Part print with two shaded views. Sizes in mm from the minimum x, y, z corner. A direction names the side the tool comes from. Give positions to 0.01 mm unless a question says otherwise; leave off trailing zeros. Loops run counter-clockwise (first coordinate to the right, second up) from the corner with the lowest first, then second, coordinate; pieces in that order, holes last. Notation, with made-up numbers: (-21, -10) -> (-11, -10) arc R11 cw to (-11, 1) -> close; hole circle Ø3 at (50.5, 51.25). An arc over 180 degrees is marked (long way). One line per question, with ' | ' between items. Start each with the question number.
(1) Slice it at D-D, the plane x = 16. Write the cut outline in (y, z).
(2) Flat gauge pins, fed straight in: pin 1 Ø2 at (x, y) = (32.5, 10) entering from +Z; pin 2 Ø2 at (x, z) = (25.72, 20.32) entering from -Y; pin 3 Ø12.5 at (x, z) = (23.5, 15) entering from -Y. Where does each tip first touch, or does it go through?
(3) Slice it at B-B, the plane z = 20.32. Write the cut outline in (x, y) (1 decimal).
(4) Drill centre lines: L1, parallel to X at y = 23.6, z = 20.32 (1 decimal); L2, parallel to X at y = 18.75, z = 1.5; L3, parallel to Y at x = 18.5, z = 13. Where is each one in solid material? Low to high. Write a range as from..to.
(5) 3-axis set-ups, long thin cutter, end or side, ignore diameter. For the marked faces 1, 2 and 3: which of +Z, -Z, +X, -X, +Y, -Y reach the whole face in a straight line?
(6) Slice it at C-C, the plane x = 29. Write the cut outline in (y, z) (1 decimal).
(7) Mould opens along X. For the marked faces 4, 5, 6 and 7 say: pulls with the +X half, pulls with the -X half, needs draft (parallel to the pull), parting line crosses it, or undercut.
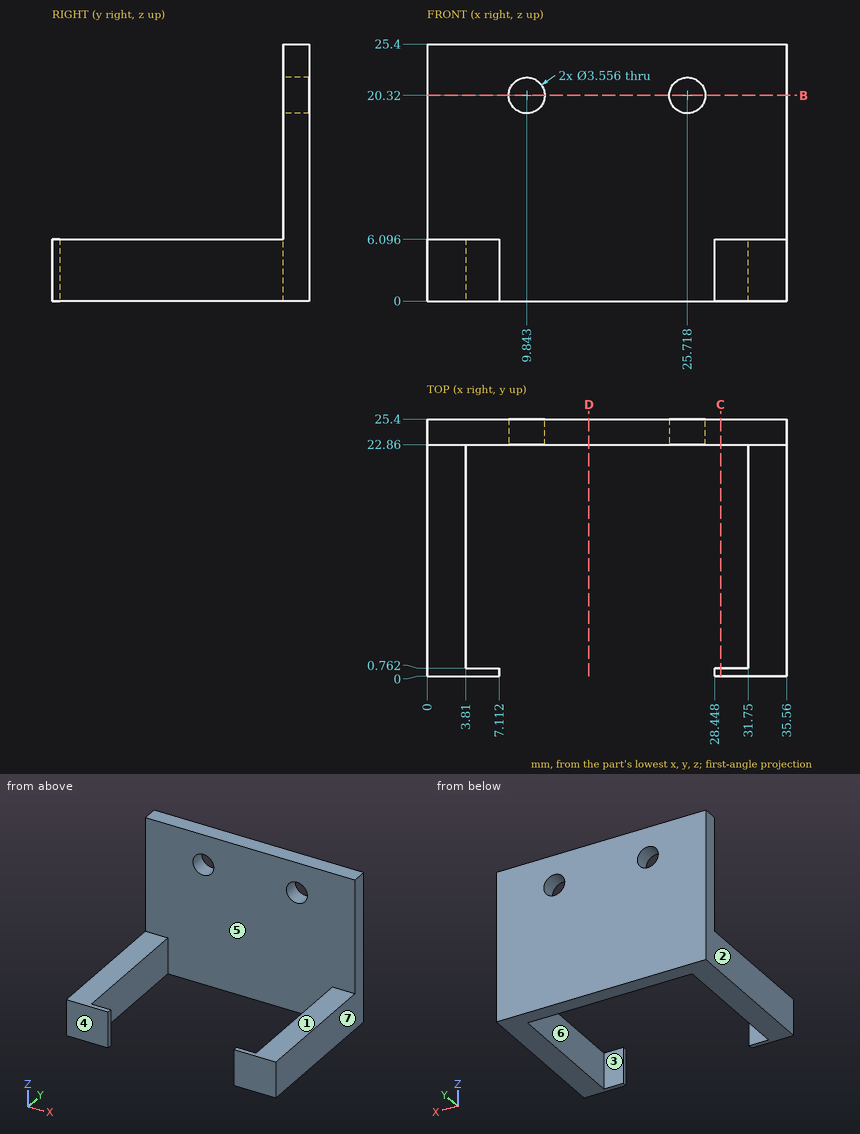
Final values:
1) outline: (22.86, 0) -> (25.4, 0) -> (25.4, 25.4) -> (22.86, 25.4) -> close
2) pin 1: z = 6.1 | pin 2: through | pin 3: y = 22.86
3) outline: (0, 22.9) -> (8.1, 22.9) -> (8.1, 25.4) -> (0, 25.4) -> close; (11.6, 22.9) -> (23.9, 22.9) -> (23.9, 25.4) -> (11.6, 25.4) -> close; (27.5, 22.9) -> (35.6, 22.9) -> (35.6, 25.4) -> (27.5, 25.4) -> close
4) L1: 0..8.1, 11.6..23.9, 27.5..35.6 | L2: 0..3.81, 31.75..35.56 | L3: 22.86..25.4
5) face 1: +Z, +X, -X, -Y | face 2: +Z, -Z, -X, +Y, -Y | face 3: +Z, -Z
6) outline: (0, 0) -> (0.8, 0) -> (0.8, 6.1) -> (0, 6.1) -> close; (22.9, 0) -> (25.4, 0) -> (25.4, 25.4) -> (22.9, 25.4) -> close
7) face 4: needs draft | face 5: undercut | face 6: undercut | face 7: pulls with the +X half
